```python
from build123d import *

# Parameters (mm, degrees)
F0_W        = 74
F0_H        = 13.15
F0_W_2      = 71
F0_H_2      = 10.15
F1_DEPTH    = 96.5
F2_DEPTH    = 95
F3_W        = 5
F3_H        = 64
F4_DEPTH    = 3
F5_T1_DEPTH = 28.15
F6_T1_DEPTH = 1.5
F7_R        = 1.49999


# Not quite as in the source:
# - a fillet or chamfer that OpenCascade refuses, or shapes differently, is made with other operations: its cross-section is extruded or revolved along the edge and cut away or added
# - a fillet or chamfer is up to 0.001 mm smaller than in the source, because OpenCascade refuses the exact size


with BuildPart() as f1:
    # F0 (on Front) → F1 (new body)
    with BuildSketch(Plane.XZ):
        Rectangle(F0_W, F0_H)
        Rectangle(F0_W_2, F0_H_2, mode=Mode.SUBTRACT)
        Rectangle(F0_W_2, F0_H_2)
    extrude(amount=F1_DEPTH)

    # F0 (on Front) → F2 (cut)
    with BuildSketch(Plane.XZ):
        Rectangle(F0_W_2, F0_H_2)
    extrude(amount=F2_DEPTH, mode=Mode.SUBTRACT)

    # F3 (on face) → F4 (cut)
    with BuildSketch(Plane.XY.offset(6.575)):
        with Locations((22.5, -47)):
            Rectangle(F3_W, F3_H)
        with Locations((-22.5, -47)):
            Rectangle(F3_W, F3_H)
    extrude(amount=-F4_DEPTH, mode=Mode.SUBTRACT)

    # F5: fillet of radius 3 on 4 edges, made by hand

    # F5_s2 → F5_t1 (cut)
    with BuildSketch(Plane.XY.offset(-14.075)):
        with BuildLine():
            ThreePointArc((37, -93.5), (36.1213203436, -95.6213203436), (34, -96.5))
            Line((34, -96.5), (37, -96.5))
            Line((37, -96.5), (37, -93.5))
        make_face()
        with BuildLine():
            ThreePointArc((-34, 0), (-36.1213203436, -0.8786796564), (-37, -3))
            Line((-37, -3), (-37, 0))
            Line((-37, 0), (-34, 0))
        make_face()
        with BuildLine():
            ThreePointArc((37, -3), (36.1213203436, -0.8786796564), (34, 0))
            Line((34, 0), (37, 0))
            Line((37, 0), (37, -3))
        make_face()
        with BuildLine():
            ThreePointArc((-34, -96.5), (-36.1213203436, -95.6213203436), (-37, -93.5))
            Line((-37, -93.5), (-37, -96.5))
            Line((-37, -96.5), (-34, -96.5))
        make_face()
    extrude(amount=F5_T1_DEPTH, mode=Mode.SUBTRACT)

    # F6: fillet of radius 3 on 8 edges, made by hand

    # F6_s2 → F6_t1 (join)
    with BuildSketch(Plane.XY.offset(5.075)):
        with BuildLine():
            ThreePointArc((25, -76), (24.1213203436, -78.1213203436), (22, -79))
            Line((22, -79), (25, -79))
            Line((25, -79), (25, -76))
        make_face()
        with BuildLine():
            ThreePointArc((23, -15), (20.8786796564, -15.8786796564), (20, -18))
            Line((20, -18), (20, -15))
            Line((20, -15), (23, -15))
        make_face()
        with BuildLine():
            ThreePointArc((25, -18), (24.1213203436, -15.8786796564), (22, -15))
            Line((22, -15), (25, -15))
            Line((25, -15), (25, -18))
        make_face()
        with BuildLine():
            ThreePointArc((23, -79), (20.8786796564, -78.1213203436), (20, -76))
            Line((20, -76), (20, -79))
            Line((20, -79), (23, -79))
        make_face()
        with BuildLine():
            ThreePointArc((-23, -79), (-20.8786796564, -78.1213203436), (-20, -76))
            Line((-20, -76), (-20, -79))
            Line((-20, -79), (-23, -79))
        make_face()
        with BuildLine():
            ThreePointArc((-25, -18), (-24.1213203436, -15.8786796564), (-22, -15))
            Line((-22, -15), (-25, -15))
            Line((-25, -15), (-25, -18))
        make_face()
        with BuildLine():
            ThreePointArc((-22, -79), (-24.1213203436, -78.1213203436), (-25, -76))
            Line((-25, -76), (-25, -79))
            Line((-25, -79), (-22, -79))
        make_face()
        with BuildLine():
            ThreePointArc((-20, -18), (-20.8786796564, -15.8786796564), (-23, -15))
            Line((-23, -15), (-20, -15))
            Line((-20, -15), (-20, -18))
        make_face()
    extrude(amount=F6_T1_DEPTH)

    # F7 (radius 1.5 in the source; OpenCascade refuses exactly that, so slightly less here)
    f7_edges = [f1.edges().sort_by_distance(p)[0] for p in [
        (0, -96.5, 6.575),
        (37, -48.25, 6.575),
        (-37, -48.25, 6.575),
        (0, -96.5, -6.575),
        (37, -48.25, -6.575),
        (-37, -48.25, -6.575),
    ]]
    fillet(f7_edges, radius=F7_R)


solid = f1.part
```
Geometry: final body of the model. Coordinates: model frame, mm. A direction names the side the tool comes from. Round coordinates to 2 decimals unless told otherwise and drop trailing zeros. Loops run counter-clockwise (first coordinate to the right, second up) from the corner with the lowest first, then second, coordinate; pieces in that order, holes last. Notation, with made-up numbers: (2, -14.5) -> (20, -14.5) arc R27 cw to (20, 8.5) -> close; hole circle Ø10 at (86.5, -13.5). An arc over 180 degrees is marked (long way). Use one line per item in the form item = value.
Item 1: Draft query along Z for faces 4 (the cylindrical face through (-20.73, -77.96, 5.81)), 5 (the flat face through (35.5, -47, 0)), 6 (the flat face through (0, -48, 6.575)). Return one class per face: released by +Z, released by -Z, zero draft, split by the parting line, or undercut.
Evaluation:
face_4 = zero draft
face_5 = undercut
face_6 = released by +Z
Item 2: Access query for faces 1 (the flat face through (0, -96.5, 0)), 2 (the flat face through (-35.5, -47, 0)), 3 (the cylindrical face through (-24.27, -77.96, 5.81)). Directions: +Z, -Z, +X, -X, +Y, -Y. A direction counts if a zero-diameter tool reaches every point of the face in a straight line with its end or side. Return the directions, or none.
Evaluation:
face_1 = +Z, -Z, +X, -X, -Y
face_2 = +Y
face_3 = +Z
Item 3: Contact query for flat-ended pins moving along their axis: pin 1 Ø0.8 at (y, z) = (-40.5, 6) entering from -X; pin 2 Ø1.5 at (x, z) = (-12.5, -4) entering from +Y. Output: stop coordinate, or through.
Evaluation:
pin_1 = -36.91
pin_2 = -95
Item 4: Cut plane A-A on y = -30.5. Output: boundary loops of the cut face in (x, z) (3 decimals).
Evaluation:
outline = (-37, -5.075) arc R1.5 ccw to (-35.5, -6.575) -> (35.5, -6.575) arc R1.5 ccw to (37, -5.075) -> (37, 5.075) arc R1.5 ccw to (35.5, 6.575) -> (25, 6.575) -> (25, 5.075) -> (35.5, 5.075) -> (35.5, -5.075) -> (-35.5, -5.075) -> (-35.5, 5.075) -> (-25, 5.075) -> (-25, 6.575) -> (-35.5, 6.575) arc R1.5 ccw to (-37, 5.075) -> close; (-20, 5.075) -> (20, 5.075) -> (20, 6.575) -> (-20, 6.575) -> close
Item 5: Cut plane B-B on y = -10.5. Output: boundary loops of the cut face in (x, z) (3 decimals), then the cut area to 3 significant figures.
Evaluation:
outline = (-37, -5.075) arc R1.5 ccw to (-35.5, -6.575) -> (35.5, -6.575) arc R1.5 ccw to (37, -5.075) -> (37, 5.075) arc R1.5 ccw to (35.5, 6.575) -> (-35.5, 6.575) arc R1.5 ccw to (-37, 5.075) -> close; hole (-35.5, -5.075) -> (35.5, -5.075) -> (35.5, 5.075) -> (-35.5, 5.075) -> close
area = 251 mm2
Item 6: Cut plane C-C on z = -2. Output: boundary loops of the cut face in (x, y), then the cut area to 3 significant figures.
Evaluation:
outline = (-37, -93.5) arc R3 ccw to (-34, -96.5) -> (34, -96.5) arc R3 ccw to (37, -93.5) -> (37, -3) arc R3 ccw to (35.5, -0.4) -> (35.5, -95) -> (-35.5, -95) -> (-35.5, -0.4) arc R3 ccw to (-37, -3) -> close
area = 389 mm2
Item 7: Material intervals for probe 1 along Z at (x, y) = (0.5, -63) (3 decimals); probe 2 along X at (y, z) = (-26.5, 3.25); probe 3 along Y at (x, z) = (-29.5, -1.5), sorted ascending.
Evaluation:
probe_1 = -6.575 to -5.075, 5.075 to 6.575
probe_2 = -37 to -35.5, 35.5 to 37
probe_3 = -96.5 to -95
